Can you work these out from the model? Positions are in its coordinate system, mm. Face numbers are marked on the shaded views. A direction names the side the tool comes from. Give positions to 0.01 mm unless a question says otherwise; leave off trailing zeros. Loops run counter-clockwise (first coordinate to the right, second up) from the corner with the lowest first, then second, coordinate; pieces in that order, holes last. Notation, with made-up numbers: (31, 7) - (60, 7) arc R28 cw to (60, 37) - close; hole circle Ø3 at (-19.75, -14). An arc over 180 degrees is marked (long way). Answer as a JSON object with one key per item and string values.
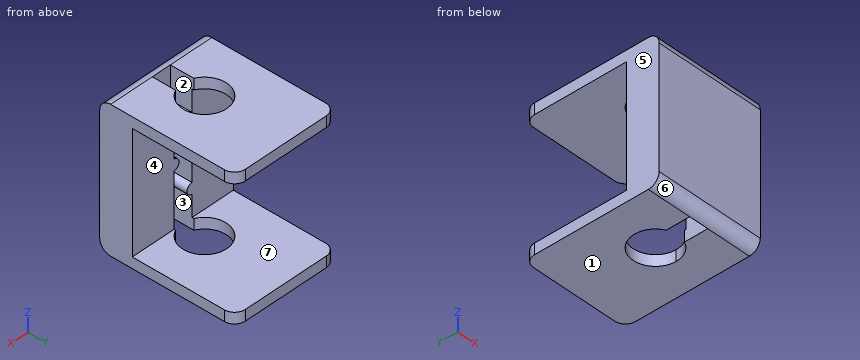
```python
from build123d import *

# Parameters (mm, degrees)
F0_W     = 4
F0_H     = 18
F1_DEPTH = 20
F3_DEPTH = 30
F5_DEPTH = 4
F6_R     = 1.99999


# Not quite as in the source:
# - a fillet or chamfer is up to 0.001 mm smaller than in the source, because OpenCascade refuses the exact size
# - a feature names something its author has since deleted; it is built from what else it names


with BuildPart() as f1:
    # F0 (on Right) → F1 (new body)
    with BuildSketch(Plane.YZ):
        Polygon((0, 26), (0, 0), (25, 0), (25, 2), (6, 2), (6, 4), (2, 4), (2, 22), (6, 22), (6, 24), (25, 24), (25, 26), align=None)
        with Locations((4, 13)):
            Rectangle(F0_W, F0_H)
    extrude(amount=F1_DEPTH)

    # F2 (on face) → F3 (cut)
    with BuildSketch(Plane.XY.offset(26)):
        with BuildLine():
            ThreePointArc((11.7568019778, 6.295455924), (9.9657604027, 5.900142972), (8.1815710291, 6.3253141525))
            Line((8.1815710291, 6.3253141525), (8.1815710291, 2))
            Line((8.1815710291, 2), (10, 2))
            Line((10, 2), (11.7568019778, 2))
            Line((11.7568019778, 2), (11.7568019778, 6.295455924))
        make_face()
        with BuildLine():
            ThreePointArc((11.7568019778, 6.295455924), (13.4650316094, 7.8082983904), (14.1, 10))
            ThreePointArc((14.1, 10), (7.8373117169, 13.4832139455), (8.1815710291, 6.3253141525))
            ThreePointArc((8.1815710291, 6.3253141525), (9.9657604027, 5.900142972), (11.7568019778, 6.295455924))
        make_face()
    extrude(amount=-F3_DEPTH, mode=Mode.SUBTRACT)

    # F4 (on face) → F5 (join)
    with BuildSketch(Plane(origin=(0, 2, 0), x_dir=(-1, 0, 0), z_dir=(0, 1, 0))):
        with BuildLine():
            ThreePointArc((-11.7568019778, 12), (-11.0496951966, 12.2928932188), (-10.7568019778, 13))
            ThreePointArc((-10.7568019778, 13), (-11.0496951966, 13.7071067812), (-11.7568019778, 14))
            Line((-11.7568019778, 14), (-11.7568019778, 12))
        make_face()
        with BuildLine():
            Line((-8.1815710291, 18), (-8.1815710291, 20))
            ThreePointArc((-8.1815710291, 20), (-9.1815710291, 19), (-8.1815710291, 18))
        make_face()
        with BuildLine():
            ThreePointArc((-7.1815710291, 19), (-7.4744642479, 19.7071067812), (-8.1815710291, 20))
            Line((-8.1815710291, 20), (-8.1815710291, 18))
            ThreePointArc((-8.1815710291, 18), (-7.4744642479, 18.2928932188), (-7.1815710291, 19))
        make_face()
        with BuildLine():
            ThreePointArc((-8.1815710291, 8), (-9.1815710291, 7), (-8.1815710291, 6))
            Line((-8.1815710291, 6), (-8.1815710291, 8))
        make_face()
    extrude(amount=F5_DEPTH)

    # F6 (radius 2 in the source; OpenCascade refuses exactly that, so slightly less here)
    f6_edges = [f1.edges().sort_by_distance(p)[0] for p in [
        (10, 0, 26),
        (10, 0, 0),
        (20, 25, 1),
        (0, 25, 1),
        (0, 25, 25),
        (20, 25, 25),
    ]]
    fillet(f6_edges, radius=F6_R)


solid = f1.part
```
1) Imagine slicing it at C-C on x = 15.75. Write out the boundary of the cut face in (y, z), and give its area (3 significant figures).
Check sheet entries:
{"outline": "(0, 2) arc R2 ccw to (2, 0) - (25, 0) - (25, 2) - (6, 2) - (6, 24) - (25, 24) - (25, 26) - (2, 26) arc R2 ccw to (0, 24) - close", "area": "230 mm2"}
2) Imagine slicing it at B-B on y = 18. Write out the boundary of the cut face in (x, z).
Check sheet entries:
{"outline": "(0, 0) - (20, 0) - (20, 2) - (0, 2) - close; (0, 24) - (20, 24) - (20, 26) - (0, 26) - close"}
3) I need wall thicknesses on L1, parallel to Z at x = 17.75, y = 11.75; L2, parallel to X at y = 10, z = 25.05; L3, parallel to Y at x = 10, z = 1.4. Which ranges of each line are inside material? Lowest first, please.
Check sheet entries:
{"L1": "0 to 2, 24 to 26", "L2": "0 to 5.9, 14.1 to 20", "L3": "0.09 to 2, 14.1 to 25"}
4) Imagine slicing it at D-D on y = 7.75. Write out the boundary of the cut face in (x, z), and give its area (3 significant figures).
Check sheet entries:
{"outline": "(0, 0) - (6.57, 0) - (6.57, 2) - (0, 2) - close; (0, 24) - (6.57, 24) - (6.57, 26) - (0, 26) - close; (13.43, 0) - (20, 0) - (20, 2) - (13.43, 2) - close; (13.43, 24) - (20, 24) - (20, 26) - (13.43, 26) - close", "area": "52.6 mm2"}
5) Imagine slicing it at A-A on x = 10. Give the number of separate pieces and of enclosed holes in the cut face, and give its area (3 significant figures).
Check sheet entries:
{"separate pieces": "3", "enclosed holes": "0", "area": "93.9 mm2"}
6) If we mould it in two halves opening along Z, with no side actions, what happens to the marked faces 5, 6 and 7? For each: released by +Z, released by -Z, zero draft, split by the parting line, or undercut.
Check sheet entries:
{"face 5": "zero draft", "face 6": "released by -Z", "face 7": "undercut"}
7) Which directions (+Z, -Z, +X, -X, +Y, -Y) give clear straight access to the entire face, cutting with the end or side of a thin tool? Please do the marked faces 1, 2, 3 and 4.
Check sheet entries:
{"face 1": "-Z, +X, -X, +Y, -Y", "face 2": "+Z", "face 3": "-Z", "face 4": "+X, -X, +Y"}
8) I'm going to push flat-ended pins straight in: P1, Ø1, axis at x = 11, z = 20, coming from the +Y side; P2, Ø10, axis at x = 13.5, z = 17.5, coming from the +Y side. Where does each tip first touch, or does it pass through?
Check sheet entries:
{"P1": "y = 2", "P2": "y = 6"}
